Verification items for the finished model (mm, model axes). A direction names the side the tool comes from. Round coordinates to 2 decimals unless told otherwise and drop trailing zeros. Order: outer loops, then holes, each group sorted by start corner. A loop starts at its lowest first (then second) coordinate and runs counter-clockwise, first axis right, second up. Notation, with made-up numbers: (6, -28) -> (32, -28) arc R20 cw to (32, 11) -> close; hole circle Ø11 at (-17.75, 22.5). An arc over 180 degrees is marked (long way). Put each result on its own line as item: value.
from build123d import *


with BuildPart() as part:
    # Sketch1 → Revolve1 (revolve)
    with BuildSketch(Plane(origin=(0, 0, 0), x_dir=(0, 0, -1), z_dir=(1, 0, 0))):
        with BuildLine():
            Line((0, 0), (0, 12.575))
            Line((0, 12.575), (-5, 12.575))
            Line((-5, 12.575), (-5, 15.75))
            Line((-5, 15.75), (-16.345423433, 15.75))
            Line((-16.345423433, 15.75), (-16.345423433, 16.5))
            Line((-16.345423433, 16.5), (-23.228752503, 16.5))
            Line((-23.228752503, 16.5), (-23.228752503, 15.75))
            Line((-23.228752503, 15.75), (-29.251665438, 15.75))
            Line((-29.251665438, 15.75), (-32.001665438, 18.5))
            Line((-32.001665438, 18.5), (-36.5, 18.5))
            Line((-36.5, 18.5), (-36.5, 17.5))
            Line((-36.5, 17.5), (-34.5, 17.5))
            Line((-34.5, 17.5), (-34.5, 16))
            Line((-34.5, 16), (-31.676037941, 13.176037941))
            Line((-31.676037941, 13.176037941), (-29.676037941, 13.176037941))
            ThreePointArc((-29.676037941, 13.176037941), (-33.951349088, 7.19510787), (-35.461393008, 0))
            Line((-35.461393008, 0), (0, 0))
        make_face()
    revolve(axis=Axis((0, 0, 35.461393008), (0, 0, -1)))


solid = part.part
Item 1: Section check D-D on z = 19.5. Record the boundary of the cut face in (x, y).
Check sheet entries:
outline: circle Ø33 at (0, 0)
Item 2: Release check for a two-part mould opening along Y. For faces 1 (the flat face through (-14.2, 7.7, 34.5)), 2 (the cylindrical face through (0.553, -12.563, 2.535)), 3 (the flat face through (-7, 11, 5)) record: +Y half, -Y half, draft (parallel to the pull), parting line (faces both ways), or undercut.
Check sheet entries:
face 1: undercut
face 2: parting line
face 3: draft
Item 3: Material ranges on L1, parallel to X at y = 0, z = 35.75; L2, parallel to X at y = 0, z = 30.9; L3, parallel to X at y = 0, z = 31.1, recorded low to high. Write a range as [from, to].
Check sheet entries:
L1: x = [-18.5, -17.5], [17.5, 18.5]
L2: x = [-17.4, -13.18], [-11.94, 11.94], [13.18, 17.4]
L3: x = [-17.6, -13.18], [-11.71, 11.71], [13.18, 17.6]
Item 4: Tool access check on faces 4 (the flat face through (-14, -11, 36.5)), 5 (the flat face through (0, 0, 0)), 6 (the conical face through (-15.54, -3.45, 29.42)), 7 (the cylindrical face through (-6.32, 15.24, 19.84)), 8 (the cylindrical face through (-10.648, -13.887, 35.486)). Record the directions out of +Z, -Z, +X, -X, +Y, -Y that give a thin tool (end or side, any length) a straight path to the whole face; none if there is none.
Check sheet entries:
face 4: +Z, +X, -X, +Y, -Y
face 5: -Z, +X, -X, +Y, -Y
face 6: none
face 7: -Z
face 8: +Z
Item 5: Gauge pin test, flat ends, axial feed: pin 1 Ø4 at (x, y) = (-10.5, -7.5) entering from +Z; pin 2 Ø1.5 at (x, z) = (4.5, 15.5) entering from +Y; pin 3 Ø16.5 at (x, y) = (2.5, 1) entering from +Z. Record the tip position at first contact, or that the pin passes through.
Check sheet entries:
pin 1: stops at z = 33.4
pin 2: stops at y = 15.3
pin 3: stops at z = 35.46
Item 6: Section check C-C on z = 28. Record the boundary of the cut face in (x, y).
Check sheet entries:
outline: circle Ø31.5 at (0, 0)
